Input: part model. Units: mm. Frame: model coordinates. Face numbers are marked on the shaded views. A direction names the side the tool comes from. Round coordinates to 2 decimals unless told otherwise and drop trailing zeros. Loops run counter-clockwise (first coordinate to the right, second up) from the corner with the lowest first, then second, coordinate; pieces in that order, holes last. Notation, with made-up numbers: (62, 2.25) -> (113, 2.25) arc R21 cw to (113, 21.25) -> close; hole circle Ø11 at (48.5, 36). An arc over 180 degrees is marked (long way). Answer as a JSON object with one key per item and string values. Group by question number.
Item 1: Section query A-A on x = 22. Return loops of the section in (y, z), and give its area (3 significant figures).
Item 2: Pin query (flat end, axial travel): pin 1 (2 mm diameter, centred on x = -29.5, z = 10.5, fed in from -Y); pin 2 (6 mm diameter, centred on x = 19, y = -34.5, fed in from +Z); pin 3 (5 mm diameter, centred on x = -27.5, z = 11.5, fed in from -Y); pin 4 (5 mm diameter, centred on y = -31.5, z = 10, fed in from -X). Return the tip coordinate at first contact, or that it passes through.
Item 3: Section query C-C on y = -20. Return loops of the section in (x, z).
Item 4: Material intervals for line 1 (Z direction, x = 11, y = 4); line 2 (X direction, y = -21.5, z = 17.5); line 3 (Y direction, x = -21.5, z = 15), sorted ascending. Write a range as [from, to].
Item 5: Section query B-B on y = 11.5. Return loops of the section in (x, z).
Item 6: Set-up query: the marked faces 3 and 4. Return all of +Z, -Z, +X, -X, +Y, -Y with unobstructed straight access to the full face (end or side cutting, diameter ignored); none if empty.
Item 7: Draft query along Y for the marked faces 1 and 2. Return one class per face: released by +Y, released by -Y, zero draft, split by the parting line, or undercut.
from build123d import *

# Parameters (mm, degrees)
F0_W     = 101.6
F0_H     = 76.2
F1_DEPTH = 19.05
F3_W     = 81.28
F3_H     = 8.89
F4_DEPTH = 31.75
F5_W     = 39.1665739621
F5_H     = 12.7
F6_DEPTH = 101.601
F7_F1_R  = 3.81
F7_F2_R  = 3.81


with BuildPart() as f1:
    # F0 (on Top) → F1 (new body)
    with BuildSketch(Plane.XY):
        with Locations((-4.0153246373, -5.6604754616)):
            Rectangle(F0_W, F0_H)
    extrude(amount=F1_DEPTH)

    # F3 (on face) → F4 (cut)
    with BuildSketch(Plane(origin=(0, 9.9172554964, 27.2474355394), x_dir=(1, 0, 0), z_dir=(0, 0.3420201433, 0.9396926208))):
        with Locations((-4.0153246373, -21.8419839543)):
            Rectangle(F3_W, F3_H)
    extrude(amount=-F4_DEPTH, mode=Mode.SUBTRACT)

    # F5 (on face) → F6 (cut, through all)
    with BuildSketch(Plane.YZ.offset(46.7846753627)):
        Polygon((-29.9731970935, 6.35), (-25.3507751184, 19.05), (-43.7604754616, 19.05), (-43.7604754616, 6.35), align=None)
        with Locations((12.8562375574, 12.7)):
            Rectangle(F5_W, F5_H)
    extrude(amount=-F6_DEPTH, mode=Mode.SUBTRACT)

    # F7: fillet of radius 3.81 on 19 edges, made by hand

    # F7_f1
    f7_f1_edges = [f1.edges().sort_by_distance(p)[0] for p in [
        (-4.0153246373, -29.9731970935, 6.35),
        (-4.0153246373, -6.7270494237, 6.35),
    ]]
    fillet(f7_f1_edges, radius=F7_F1_R)

    # F7_f2
    f7_f2_edges = [f1.edges().sort_by_distance(p)[0] for p in [
        (-4.0153246373, -25.3507751184, 19.05),
        (-4.0153246373, -6.7270494237, 19.05),
        (46.7846753627, -38.2007316379, 6.35),
        (-4.0153246373, -43.7604754616, 6.35),
        (-54.8153246373, -38.2007316379, 6.35),
        (-54.8153246373, 14.7612375574, 6.35),
        (-4.0153246373, 32.4395245384, 6.35),
        (46.7846753627, 14.7612375574, 6.35),
        (46.7846753627, 32.4395245384, 3.175),
        (46.7846753627, -43.7604754616, 3.175),
        (-54.8153246373, -43.7604754616, 3.175),
        (-54.8153246373, -27.2057670236, 13.953451627),
        (-54.8153246373, -6.7270494237, 14.605),
        (46.7846753627, -27.2057670236, 13.953451627),
        (46.7846753627, -16.038912271, 19.05),
        (-54.8153246373, -16.038912271, 19.05),
        (-54.8153246373, 32.4395245384, 3.175),
        (46.7846753627, -30.4556615916, 7.0390307113),
        (-54.8153246373, -5.61112626, 7.4659231637),
        (-54.8153246373, -30.4556615916, 7.0390307113),
        (46.7846753627, -5.61112626, 7.4659231637),
    ]]
    fillet(f7_f2_edges, radius=F7_F2_R)


solid = f1.part
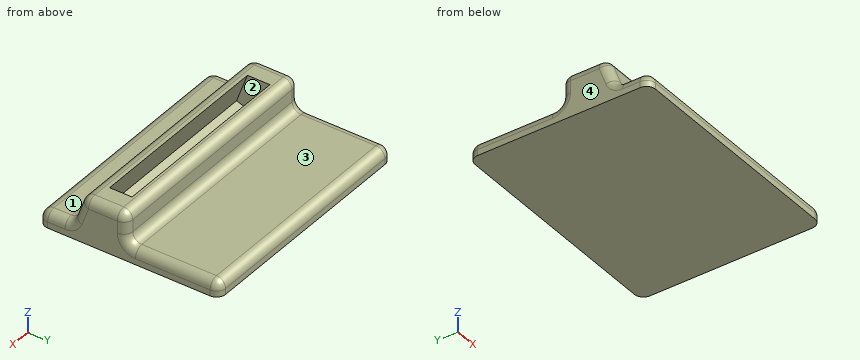
Solved:
{
 "1": {"outline": "(-43.76, 0) -> (32.44, 0) -> (32.44, 2.54) arc R3.81 ccw to (28.63, 6.35) -> (-2.92, 6.35) arc R3.81 cw to (-6.73, 10.16) -> (-6.73, 15.24) arc R3.81 ccw to (-10.54, 19.05) -> (-11.58, 19.05) -> (-17.29, 3.36) -> (-25.64, 6.4) -> (-21.04, 19.05) -> (-22.68, 19.05) arc R3.81 ccw to (-26.26, 16.54) -> (-29.06, 8.86) arc R3.81 cw to (-32.64, 6.35) -> (-39.95, 6.35) arc R3.81 ccw to (-43.76, 2.54) -> close", "area": "609 mm²"},
 "2": {"pin 1": "y = -28.83", "pin 2": "z = 6.52", "pin 3": "y = -29.01", "pin 4": "through"},
 "3": {"outline": "(-54.82, 0) -> (46.78, 0) -> (46.78, 15.24) arc R3.81 ccw to (42.97, 19.05) -> (36.62, 19.05) -> (36.62, 4.35) -> (-44.66, 4.35) -> (-44.66, 19.05) -> (-51.01, 19.05) arc R3.81 ccw to (-54.82, 15.24) -> close"},
 "4": {"line 1": "[0, 6.35]", "line 2": "[-54.07, -44.66], [36.62, 46.04]", "line 3": "[-26.82, -22.51], [-13.05, -6.73]"},
 "5": {"outline": "(-54.82, 0) -> (46.78, 0) -> (46.78, 2.54) arc R3.81 ccw to (42.97, 6.35) -> (-51.01, 6.35) arc R3.81 ccw to (-54.82, 2.54) -> close"},
 "6": {"face 3": "+Z, +X, -X, +Y", "face 4": "+Z, -Z, -X, +Y, -Y"},
 "7": {"face 1": "zero draft", "face 2": "undercut"}
}
